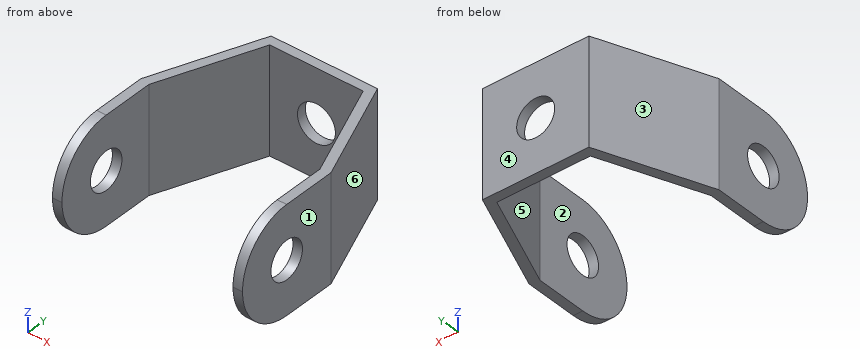
```python
from build123d import *

# Parameters (mm, degrees)
ESBO_O1_W                  = 50
ESBO_O1_H                  = 56
RESSALTO_EXTRUS_O1_DEPTH   = 28
CORTE_EXTRUS_O1_DEPTH      = 28
CORTE_EXTRUS_O7_DEPTH      = 28
CORTE_EXTRUS_O7_DEPTH_BACK = 28
ESBO_O7_R                  = 5
CORTE_EXTRUS_O8_DEPTH      = 64.780874876
ESBO_O8_R                  = 5
CORTE_EXTRUS_O9_DEPTH      = 68.416615163
FILETE7_R                  = 14
FILETE8_R                  = 14


with BuildPart() as part:
    # Esboço1 → Ressalto-extrusão1 (new body)
    with BuildSketch(Plane.XY):
        Rectangle(ESBO_O1_W, ESBO_O1_H)
    extrude(amount=RESSALTO_EXTRUS_O1_DEPTH)

    # Esboço5 → Corte-extrusão1 (cut)
    with BuildSketch(Plane.XY.offset(28)):
        Polygon((-22.5, -0.473458617), (-22.5, -28), (22.5, -28), (22.5, -0.473458617), (12.296141258, 25.5), (0, 25.5), (-12.296141258, 25.5), align=None)
    extrude(amount=-CORTE_EXTRUS_O1_DEPTH, mode=Mode.SUBTRACT)

    # Esboço2 → Corte-extrusão7 (cut, two sides: drawn at the far end of the back side and taken through both)
    with BuildSketch(Plane.XY.offset(-CORTE_EXTRUS_O7_DEPTH_BACK)):
        Polygon((-14, 28), (-25, 28), (-25, 0), align=None)
        Polygon((25, 0), (25, 28), (14, 28), align=None)
    extrude(amount=CORTE_EXTRUS_O7_DEPTH + CORTE_EXTRUS_O7_DEPTH_BACK, mode=Mode.SUBTRACT)

    # Esboço7 → Corte-extrusão8 (cut, through all)
    with BuildSketch(Plane.ZY.offset(25)):
        with Locations(Location((14, -14, 0), (0, 0, 270))):
            Circle(ESBO_O7_R)
    extrude(amount=-CORTE_EXTRUS_O8_DEPTH, mode=Mode.SUBTRACT)

    # Esboço8 → Corte-extrusão9 (cut, through all)
    with BuildSketch(Plane(origin=(0, 28, 0), x_dir=(1, 0, 0), z_dir=(0, 1, 0))):
        with Locations(Location((0, -14, 0), (0, 0, 270))):
            Circle(ESBO_O8_R)
    extrude(amount=-CORTE_EXTRUS_O9_DEPTH, mode=Mode.SUBTRACT)

    # Filete7
    filete7_edges = [part.edges().sort_by_distance(p)[0] for p in [
        (-23.75, -28, 0),
        (-23.75, -28, 28),
    ]]
    fillet(filete7_edges, radius=FILETE7_R - 0.0001)  # a hair under: the kernel refuses the full size

    # Filete8
    filete8_edges = [part.edges().sort_by_distance(p)[0] for p in [
        (23.75, -28, 28),
        (23.75, -28, 0),
    ]]
    fillet(filete8_edges, radius=FILETE8_R - 0.0001)  # a hair under: the kernel refuses the full size


solid = part.part
```
Work out the finished part from the listing and answer in its coordinate system (mm). Face numbers are marked on the shaded views. A direction names the side the tool comes from. Coordinates: 2 decimals unless noted, no trailing zeros. Order: outer loops, then holes, each group sorted by start corner. A loop starts at its lowest first (then second) coordinate and runs counter-clockwise, first axis right, second up. Notation, with made-up numbers: M -29.5,-39.5 L -24.5,-39.5 A16 ccw -24.5,-20.5 Z; hole C 88.5,65 d3. An arc over 180 degrees is marked long. Use CSV: the item, a comma, the result in double quotes.
1) Section B-B on x = 0 is taken. Write down the section's boundary in (y, z).
Worked out:
outline,"M 25.5,0 L 28,0 L 28,9 L 25.5,9 Z; M 25.5,19 L 28,19 L 28,28 L 25.5,28 Z"
2) Determine the mould class of the marked faces 3, 4, 5 and 6 for opening direction X: released by +X, released by -X, zero draft, split by the parting line, or undercut.
Worked out:
face 3,"released by -X"
face 4,"zero draft"
face 5,"undercut"
face 6,"released by +X"
3) Section C-C on z = 17 is taken. Write down the section's boundary in (x, y).
Worked out:
outline,"M -25,-27.67 L -22.5,-27.67 L -22.5,-18 L -25,-18 Z; M -25,-10 L -22.5,-10 L -22.5,-0.47 L -12.3,25.5 L -4,25.5 L -4,28 L -14,28 L -25,0 Z; M 4,25.5 L 12.3,25.5 L 22.5,-0.47 L 22.5,-10 L 25,-10 L 25,0 L 14,28 L 4,28 Z; M 22.5,-27.67 L 25,-27.67 L 25,-18 L 22.5,-18 Z"
4) Section A-A on y = -8 is taken. Write down the section's boundary in (x, z), plus the area to 3 significant figures.
Worked out:
outline,"M -25,0 L -22.5,0 L -22.5,28 L -25,28 Z; M 22.5,0 L 25,0 L 25,28 L 22.5,28 Z"
area,"140 mm^2"
5) Section D-D on y = -15 is taken. Write down the section's boundary in (x, z).
Worked out:
outline,"M -25,0.04 L -22.5,0.04 L -22.5,9.1 L -25,9.1 Z; M -25,18.9 L -22.5,18.9 L -22.5,27.96 L -25,27.96 Z; M 22.5,0.04 L 25,0.04 L 25,9.1 L 22.5,9.1 Z; M 22.5,18.9 L 25,18.9 L 25,27.96 L 22.5,27.96 Z"
6) Consider line 1 (X direction, y = -22.5, z = 13); line 2 (Z direction, x = 24, y = -14); line 3 (X direction, y = 17.5, z = 21.5) (3 decimals). Determine where each line is inside the solid, lowest interval first. Write a range as [from, to].
Worked out:
line 1,"x = [-25, -22.5], [22.5, 25]"
line 2,"z = [0, 9], [19, 28]"
line 3,"x = [-18.125, -15.439], [15.439, 18.125]"
7) Flat-ended cylindrical pins translate along their axes: pin 1 Ø2 at (y, z) = (8.5, 4) entering from +X; pin 2 Ø8 at (x, z) = (3.5, 14.5) entering from -Y; pin 3 Ø9 at (y, z) = (-14, 14) entering from +X. Find the tip coordinate at first contact, or state that the pin passes through.
Worked out:
pin 1,"stops at x = 22.05"
pin 2,"stops at y = 25.5"
pin 3,"passes through"
8) For the marked faces 1 and 2, determine the directions among +Z, -Z, +X, -X, +Y, -Y from which every point of the face is accessible in a straight line to the end or side of a thin tool.
Worked out:
face 1,"+Z, -Z, +X, +Y, -Y"
face 2,"+Z, -Z, -Y"
